Autodesk Inventor part; units mm, degrees
ref_plane "Plano de trabajo2" through (0, 177.05, 0) normal (0, 1, 0) x (-1, 0, 0)
ref_plane "YZ Plane" through (0, 0, 0) normal (1, 0, 0) x (0, 1, 0)
ref_plane "XY Plane" through (0, 0, 0) normal (0, 0, 1) x (1, 0, 0)
sketch "Boceto1" plane through (0, 0, 0) normal (1, 0, 0) x (0, 1, 0)
  circle A0 centre (0, 0) radius 5
  line L0 (0, 0) -> (0, 6)
  line L1 (0, 6) -> (-4, 6)
  line L2 (-5, 5) -> (-5, 0)
  line L3 (0, 6) -> (181.05, 6)
  line L4 (181.05, 6) -> (187.5, 6)
  line L5 (187.5, 6) -> (189.65, 6)
  line L6 (190.65, 5) -> (190.65, -1)
  line L7 (189.65, -2) -> (4.5826, -2)
  arc A1 (-4, 6) -> (-5, 5) centre (-4, 5) ccw
  arc A2 (190.65, 5) -> (189.65, 6) centre (189.65, 5) ccw
  arc A3 (189.65, -2) -> (190.65, -1) centre (189.65, -1) ccw
  line L8 (3.5707, -3.5) -> (-3.5707, -3.5)
  point P0 (-5, 6)
  point P1 (190.65, 6)
  point P2 (190.65, -2)
  dimension "d0" = 10
  dimension "d1" = 6
  dimension "d2" = 5
  dimension "d3" = 181.05
  dimension "d4" = 6.45
  dimension "d5" = 3.15
  dimension "d6" = 8
  dimension "d7" = 1
  dimension "d8" = 1
  dimension "d45" = 1.5
extrude "Extrusión1" add sketch "Boceto1" along normal mid plane 8 contours A0 L8 | L2 A1 L1 L0 A0 | L0 L3 L4 L5 A2 L6 A3 L7 A0 picked at (0, -0.6667)
fillet "Empalme1" radius 1 18 edges at (-4, 190.3571, 5.7071) (-4, 190.65, 2) (-4, 190.3571, -1.7071) (-4, 97.1163, -2) (-4, -4.7071, 5.7071) (-4, -5, 2.5) (-4, -4.6289, -1.8903) (-4, 4.1451, -2.7962) (-4, 92.825, 6) (4, -4.7071, 5.7071) (4, -5, 2.5) (4, -4.6289, -1.8903) (4, 4.1451, -2.7962) (4, 190.3571, 5.7071) (4, 190.65, 2) (4, 190.3571, -1.7071) (4, 97.1163, -2) (4, 92.825, 6)
sketch "Boceto2" plane through (-4, 0, 0) normal (-1, 0, 0) x (0, 0, 1)
  circle A0 centre (0, 0) radius 5.5
  line L0 (4.7631, 2.75) -> (-2, 14.4641)
  line L1 (-2, 189.65) -> (-2, 4.5826)
  line L2 (5.5, 0) -> (5.5, -5.5)
  line L3 (0, -5) -> (5, -5)
  line L4 (0, -5.5) -> (5.5, -5.5)
  line L5 (-2, 14.4641) -> (-2, 5.1235)
  dimension "d12" = 11
  dimension "d13" = 30
extrude "Extrusión2" cut sketch "Boceto2" against normal blind 2.5
sketch "Boceto3" plane through (0, 0, 0) normal (0, 0, 1) x (1, 0, 0)
  line L0 (-3, 190.65) -> (3, 190.65)
  line L1 (0, 190.65) -> (0, 181.05)
  line L2 (1.4, 190.65) -> (1.4, 181.05)
  line L3 (-1.4, 190.65) -> (-1.4, 181.05)
  line L4 (1.4, 190.65) -> (-1.4, 190.65)
  line L5 (0, 181.05) -> (1.4, 181.05)
  line L6 (0, 181.05) -> (-1.4, 181.05)
  point P0 (0, 0)
  dimension "d16" = 9.6
  dimension "d17" = 1.4
  dimension "d18" = 1.4
extrude "Extrusión3" cut sketch "Boceto3" along normal mid plane 16
fillet "Empalme4" radius 1 2 edges at (-1.4, 181.05, 2) (1.4, 181.05, 2)
sketch "Boceto11" plane through (0, 0, 0) normal (1, 0, 0) x (0, 1, 0)
  line L0 (0, 0) -> (0, 6)
  line L1 (0, 6) -> (181.05, 6)
  line L2 (189.65, 6) -> (-4, 6)
  line L3 (181.05, 6) -> (187.5, 6)
  line L4 (187.5, 6) -> (187.5, 0.55)
  circle A0 centre (187.5, 0.55) radius 1.15
  dimension "d66" = 6
  dimension "d67" = 181.05
  dimension "d68" = 6.45
  dimension "d69" = 5.45
  dimension "d70" = 2.3
extrude "Extrusión9" cut sketch "Boceto11" along normal through all both and the other way through all
sketch "Boceto6" plane through (0, 0, 0) normal (0, 0, 1) x (1, 0, 0)
  line L0 (0, 0) -> (-1.5, 0)
  line L1 (-1.5, 0) -> (-1.5, -3)
  line L2 (-1.5, -5) -> (-1.5, 4.5826)
  line L3 (-1.5, -3) -> (-4.5, -3)
  line L4 (-1.5, 0) -> (-9.5, 0)
  line L5 (-4.5, -3) -> (-4.5, -3.5)
  line L6 (-9.5, 0) -> (-9.5, -2.3732)
  line L7 (-9.5, -2.3732) -> (-4.5, -3.5)
  dimension "d27" = 1.5
  dimension "d28" = 3
  dimension "d29" = 3
  dimension "d30" = 8
  dimension "d31" = 0.5
  dimension "d32" = 2.3732
revolve "Revolución1" add sketch "Boceto6" angle 360 about axis through (-1.5, 0, 0) along (-1, 0, 0)
sketch "Boceto7" plane through (0, 0, 0) normal (0, 0, 1) x (1, 0, 0)
  line L0 (0, 0) -> (-1.5, 0)
  line L1 (-1.5, 0) -> (-4.5, 0)
  line L2 (-4.5, 0) -> (-9.5, 0)
  line L3 (-9.5, 0) -> (-9.5, -1)
  line L4 (-9.5, 2.3732) -> (-9.5, -2.3732)
  line L5 (-9.5, -1) -> (-2.5, -1)
  line L6 (-2.5, -1) -> (-2.5, 1)
  line L7 (-2.5, 1) -> (-9.5, 1)
  line L8 (-9.5, 1) -> (-9.5, 0)
  point P0 (-9.5, 1)
  dimension "d34" = 1.5
  dimension "d35" = 3
  dimension "d36" = 5
  dimension "d37" = 1
  dimension "d38" = 7
  dimension "d39" = 2
extrude "Extrusión5" cut sketch "Boceto7" along normal mid plane 7
fillet "Empalme2" radius 1 2 edges at (-2.5, -1, 0) (-2.5, 1, 0)
ref_plane "Plano de trabajo2" through (0, 177.05, 0) normal (0, 1, 0) x (-1, 0, 0)
sketch "Boceto8" plane through (0, 177.05, 0) normal (0, 1, 0) x (-1, 0, 0)
  line L0 (0, 0) -> (0, 2)
  line L1 (16, 18) -> (-16, 18)
  line L2 (-16, 18) -> (-16, -14)
  line L3 (-16, -14) -> (16, -14)
  line L4 (16, -14) -> (16, 18)
  line L5 (16, 18) -> (-16, -14) construction
  line L6 (-16, 18) -> (16, -14) construction
  point P0 (0, 0)
  dimension "d49" = 2
  dimension "d50" = 32
  dimension "d51" = 32
  dimension "d78" = 0
extrude "Extrusión6" cut sketch "Boceto8" against normal blind 362.1
sketch "Boceto9" plane through (0, 177.05, 0) normal (0, -1, 0) x (-1, 0, 0)
  line L0 (3, -6) -> (-3, -6)
  line L1 (0, 0) -> (0, -2)
  circle A0 centre (0, -2) radius 2.5
  point P0 (0, 0)
  point P1 (-2.6, -6)
  dimension "d55" = 2
  dimension "d56" = 5
  dimension "d79" = 0
  dimension "d80" = 0
extrude "Extrusión7" add sketch "Boceto9" along normal blind 44
sketch "Boceto10" plane through (0, 177.05, 0) normal (0, -1, 0) x (-1, 0, 0)
  circle A0 centre (0, -2) radius 2.5
  circle A1 centre (0, -2) radius 3
  point P0 (0, 0)
  dimension "d59" = 6
extrude "Extrusión8" add sketch "Boceto10" along normal blind 2 contours A0 | A1
fillet "Empalme3" radius 1 1 edges at (2.5, 175.05, 2)
equation "\"d0\" = width_r3"
equation "\"d1\" = 0.5 * width_r3 + offset"
equation "\"d3\" = lenght_body_link - 0.5 * width_r3"
equation "\"d4\" = shaft_y"
equation "\"d45\" = 1.5 * offset"
equation "\"d9\" = width_link"
equation "\"d12\" = width_r3 + offset"
equation "\"d14\" = 0.5 * width_link - 0.5 * t_thikness"
equation "\"d16\" = 0.5 * Djoint_shaft + 2 * offset + shaft_y"
equation "\"d17\" = 0.25 * offset + 0.5 * wire_D"
equation "\"d18\" = 0.25 * offset + 0.5 * wire_D"
equation "\"d19\" = 2 * width_link"
equation "\"d63\" = offset"
equation "\"d27\" = 0.5 * t_thikness"
equation "\"d28\" = 0.5 * sj_diam_shaft"
equation "\"d29\" = t_thikness"
equation "\"d30\" = t_thikness + sj_head_height"
equation "\"d31\" = 0.5 * sj_head_D - 0.5 * sj_diam_shaft"
equation "\"d32\" = 0.5 * sj_head_d"
equation "\"d34\" = 0.5 * t_thikness"
equation "\"d35\" = t_thikness"
equation "\"d36\" = sj_head_height"
equation "\"d37\" = 0.5 * sj_groove"
equation "\"d38\" = sj_groove_deep"
equation "\"d39\" = sj_groove"
equation "\"d40\" = sj_head_D"
equation "\"d46\" = 0.5 * sj_groove"
equation "\"d56\" = spring_int_d - offset"
equation "\"d59\" = spring_int_d"
equation "\"d60\" = thikness"
equation "\"d62\" = offset"
equation "\"offset\" = 1"
equation "\"wire_D\" = 2.3"
equation "\"width_link\" = 8"
equation "\"Djoint_shaft\" = 2.3"
equation "\"shaft_x\" = 1.45"
equation "\"shaft_y\" = 6.45"
equation "\"lenght_body_link\" = 186.05"
equation "\"m2_theta3f\" = -60deg"
equation "\"width_r3\" = 10"
equation "\"t_thikness\" = 3"
equation "\"sj_diam_shaft\" = 6"
equation "\"sj_groove\" = 2"
equation "\"sj_groove_deep\" = 7"
equation "\"sj_head_D\" = 7"
equation "\"sj_head_d\" = 4.7464"
equation "\"sj_head_height\" = 5"
equation "\"thikness\" = 2"
equation "\"spring_int_d\" = 6"
equation "\"spring_lenght\" = 28"
equation "\"r1\" = 5.55"
equation "\"r2o\" = 59.75"
equation "\"delta_y\" = 6"
equation "\"wire_d\" = 1"
equation "\"width_ang_spring\" = 5"
equation "\"spring_int_diam\" = 8.5"
equation "\"spring_ext_diam\" = 10.5"
equation "\"r3\" = 8.25"
equation "\"r3R\" = 4.75"
equation "\"r3T\" = 6.74537"
equation "\"alpha\" = 54.847297deg"
equation "\"alpha2\" = 270deg"
equation "\"theta3_recogido\" = 305.152703deg"
equation "\"delta_theta_3\" = 45deg"
equation "\"joint_width\" = 12"
equation "\"joint_radius\" = 7.75"
equation "\"shaft_width\" = 15"
equation "\"shaft_joint_diameter\" = 7.75"
equation "\"separation_space\" = 0.5"
equation "\"height_finger\" = 42"
equation "\"cell_screw_head_diameter\" = 4"
equation "\"cell_screw_diameter\" = 2"
equation "\"cell_space\" = 2"
equation "\"cell_width\" = 6"
equation "\"cell_theta_position\" = 60deg"
equation "\"cell_thikness\" = 1"
equation "\"cell_lenght\" = 37"
equation "\"cell_z_space\" = 5"
equation "\"Dt\" = 1.05949"
equation "\"lenght_bar_support\" = 201.65"
equation "\"wire_spring_d\" = 1"
equation "\"trigger_offset\" = 2"
equation "\"m2_theta2o\" = 107deg"
equation "\"m2_r2\" = 28"
equation "\"e\" = 9"
equation "\"So\" = 17"
equation "\"m2_theta3o\" = -30deg"
equation "\"m2_r3\" = 19.75"
equation "\"m2_delta_theta1\" = 15deg"
equation "\"trigger_thumb_lenght\" = 6"
equation "\"width_r12\" = 8"
equation "\"m2_r1\" = 25.2"
equation "\"r3_thikness\" = 3.5"
equation "\"tg_width\" = 4"
equation "\"pivot_screw_d\" = 4"
equation "\"pivot_diameter\" = 7"
equation "\"sf_lenght\" = 9.5"
equation "\"sf_base\" = 3"
equation "\"sf_head_height\" = 3"
equation "\"sf_head_width\" = 4.5"
equation "\"sf_head_offset\" = 0.25"
equation "\"sf_head_grip_width\" = 2"
equation "\"sf_head_angle\" = 45deg"
equation "\"sf_thikness\" = 5"
equation "\"screw_Dhead\" = 8"
equation "\"screw_d\" = 4"
equation "\"screw_lenght\" = 12"
equation "\"screwJ_base_D\" = 9"
equation "\"screwJ_top_D\" = 13"
equation "\"gj_D\" = 6"
equation "\"gj_d\" = 4"
equation "\"gj_out_section\" = 6"
equation "\"agarradera_theta\" = 60deg"
equation "\"agarradera_width\" = 4"
equation "\"sfbox_theta1\" = 60deg"
equation "\"sfbox_theta2\" = 45deg"
equation "\"position\" = 39.13077"
equation "\"fat_width_slider\" = 2"
equation "\"sfbox_tip_width\" = 2.5"
equation "\"flex_separation_theta\" = 60deg"
equation "\"sf_flex_separation\" = 38.66667"
equation "\"ext_width_slider\" = 3.5"
equation "\"sf_box_width\" = 1.5"
equation "\"slim_width_slider\" = 1.5"
equation "\"sfbox_width\" = 1.5"
equation "\"int_width_slider\" = 2"
equation "\"box_fat_slider_lenght\" = 67"
equation "\"box_slim_slider_lenght\" = 116"
equation "\"thikness_box\" = 1.5"
equation "\"box_in_height\" = 35"
equation "\"box_in_width\" = 72"
equation "\"box_in_deep\" = 77"
equation "\"agarradera_position\" = 82.13077"
properties part number "Eslabón conector M1" material "Plástico PPS"
Can you work these out from the model? Positions are in its coordinate system, mm. A direction names the side the tool comes from. Give positions to 0.01 mm unless a question says otherwise; leave off trailing zeros. Write each loop counter-clockwise with the first axis right and the second up, starting at its lowest first coordinate (ties: lowest second). Pieces come first, ordered by that corner, then holes. Notation, with made-up numbers: (-15.5, 85) -> (27.5, 85) arc R18 cw to (27.5, 103) -> close; hole circle Ø6 at (16.25, -23). An arc over 180 degrees is marked (long way). Write item = value, one per line.
(1) I'm going to push flat-ended pins straight in: P1, Ø2, axis at x = 0, y = 154, coming from the -Z side; P2, Ø2, axis at y = 187.5, z = 0.55, coming from the +X side; P3, Ø1.5, axis at y = 147.5, z = 4.5, coming from the -X side; P4, Ø2, axis at x = -0.5, y = 170.5, coming from the +Z side. Where does each tip first touch, or does it pass through?
Worked out:
P1 = -0.5
P2 = through
P3 = -1.79
P4 = 4.5
(2) Thinking about a two-plate mould opening in Z: for faces 1 (the face through (2.21, 176.06, 4.03)), 2 (the face through (2.682, 188.597, 0.205)), 3 (the face through (-4, 183, 2)), which applies, released by +Z, released by -Z, zero draft, split by the parting line, or undercut?
Worked out:
face_1 = split by the parting line
face_2 = undercut
face_3 = zero draft
(3) Suppose I cut it at A-A on y = 187.5. Write out the boundary of the cut face in (x, z), then the cut area to 3 significant figures.
Worked out:
outline = (-4, -1) arc R1 ccw to (-3, -2) -> (-1.4, -2) -> (-1.4, -0.6) -> (-4, -0.6) -> close; (-4, 1.7) -> (-1.4, 1.7) -> (-1.4, 6) -> (-3, 6) arc R1 ccw to (-4, 5) -> close; (1.4, -2) -> (3, -2) arc R1 ccw to (4, -1) -> (4, -0.6) -> (1.4, -0.6) -> close; (1.4, 1.7) -> (4, 1.7) -> (4, 5) arc R1 ccw to (3, 6) -> (1.4, 6) -> close
area = 28.8 mm^2
(4) Suppose I cut it at C-C on y = 171.5. Write out the boundary of the cut face in (x, z), then the cut area to 3 significant figures.
Worked out:
outline = circle Ø5 at (0, 2)
area = 19.6 mm^2
(5) For faces 4 (the face through (-1.115, 181.351, 2.056)), 5 (the face through (3.699, 183.438, 5.715)), 6 (the face through (-2, 177.05, 5)), which set-ups out of +Z, -Z, +X, -X, +Y, -Y let a thin tool reach every point of the face, with its end or its side?
Worked out:
face_4 = +Z, -Z, +Y
face_5 = +Z, +X, +Y, -Y
face_6 = -Y
(6) Suppose I cut it at B-B on z = 0.55. Count the separate pieces of the cut face and the enclosed holes in it, then the cut area to 3 significant figures.
Worked out:
separate_pieces = 3
enclosed_holes = 0
area = 252 mm^2
(7) I need wall thicknesses on probe 1 along Z at (x, y) = (-2.7, 187.5); probe 2 along Y at (x, z) = (-2.75, 0.5); probe 3 along Y at (x, z) = (0.5, 5). Which ranges of each line are inside material? Lowest first, please. Write a range as from..to.
Worked out:
probe_1 = -2..-0.6, 1.7..6
probe_2 = 177.05..186.35, 188.65..190.65
probe_3 = 177.05..181.06
